CAD build for the part. Positions are in the model's coordinates, mm. A direction names the side the tool comes from. Round coordinates to 2 decimals unless told otherwise and drop trailing zeros. Order: outer loops, then holes, each group sorted by start corner. A loop starts at its lowest first (then second) coordinate and runs counter-clockwise, first axis right, second up. Notation, with made-up numbers: M 58,-16 L 81,-16 A23 cw 81,3 Z; hole C 56,-6.5 d7. An arc over 180 degrees is marked long. Put each result on its own line as item: value.
```python
from build123d import *

# Parameters (mm, degrees)
SKETCH4_W              = 63.5
SKETCH4_H              = 44.45
BASE_FLANGE1_DEPTH     = 1.905
SKETCHED_START         = -31.75
SKETCHED_BEND3_DEPTH   = 63.5
SKETCHED_BEND3_2_DEPTH = 63.5
CUT_EXTRUDE2_REACH     = 44.696
SKETCH20_R             = 2


# Read off the part's stored shape, not the designer's step: Sketched Bend3
# Sheet-metal steps are written as plain solids
with BuildPart() as part:
    # Sketch4 → Base-Flange1 (new body)
    with BuildSketch(Plane(origin=(0, 0, 0), x_dir=(0, 0, -1), z_dir=(1, 0, 0))):
        Rectangle(SKETCH4_W, SKETCH4_H)
    extrude(amount=-BASE_FLANGE1_DEPTH)

    # Sketched Bend3 outline → Sketched Bend3 (cut)
    with BuildSketch(Plane.XY.offset(SKETCHED_START)):
        with BuildLine():
            ThreePointArc((0, -13.357223013), (-1.375727285, -12.406629491), (-1.905, -10.8204))
            Line((-1.905, -10.8204), (-1.905, -22.225))
            Line((-1.905, -22.225), (0, -22.225))
            Line((0, -22.225), (0, -13.357223013))
        make_face()
        with BuildLine():
            Line((-1.905, 22.225), (-1.905, 10.8204))
            ThreePointArc((-1.905, 10.8204), (-1.375727285, 12.406629491), (0, 13.357223013))
            Line((0, 13.357223013), (0, 22.225))
            Line((0, 22.225), (-1.905, 22.225))
        make_face()
    extrude(amount=SKETCHED_BEND3_DEPTH, mode=Mode.SUBTRACT)

    # Sketched Bend3 2 outline → Sketched Bend3 2 (add)
    with BuildSketch(Plane.XY.offset(SKETCHED_START)):
        with BuildLine():
            Line((0, -10.8204), (0, -13.357223013))
            ThreePointArc((0, -13.357223013), (0.364592683, -13.435674577), (0.7366, -13.462))
            Line((0.7366, -13.462), (9.487967924, -13.462))
            Line((9.487967924, -13.462), (9.487967924, -11.557))
            Line((9.487967924, -11.557), (0.7366, -11.557))
            ThreePointArc((0.7366, -11.557), (0.215745145, -11.341254855), (0, -10.8204))
        make_face()
        with BuildLine():
            ThreePointArc((0.7366, 13.462), (0.364592683, 13.435674577), (0, 13.357223013))
            Line((0, 13.357223013), (0, 10.8204))
            ThreePointArc((0, 10.8204), (0.215745145, 11.341254855), (0.7366, 11.557))
            Line((0.7366, 11.557), (9.487967924, 11.557))
            Line((9.487967924, 11.557), (9.487967924, 13.462))
            Line((9.487967924, 13.462), (0.7366, 13.462))
        make_face()
    extrude(amount=SKETCHED_BEND3_2_DEPTH)

    # Cut-Extrude2: up to this face of the body (flat: up to its plane)
    cut_extrude2_end = Plane(part.part.faces().sort_by_distance((5.112283962, -13.462, 0))[0])
    # Sketch20 → Cut-Extrude2 (cut, up to the picked face)
    with BuildSketch(Plane(origin=(0, 13.462, 0), x_dir=(1, 0, 0), z_dir=(0, 1, 0)), mode=Mode.PRIVATE) as cut_extrude2_sk1:
        with Locations(Location((5.08, 0, 0), (0, 0, 180))):
            Circle(SKETCH20_R)
    cut_extrude2_tool1 = split(extrude(cut_extrude2_sk1.sketch, amount=-CUT_EXTRUDE2_REACH, mode=Mode.PRIVATE), bisect_by=cut_extrude2_end, keep=Keep.BOTH, mode=Mode.PRIVATE)
    # Sketch20 → Cut-Extrude2 (cut, up to the picked face)
    with BuildSketch(Plane(origin=(0, 13.462, 0), x_dir=(1, 0, 0), z_dir=(0, 1, 0)), mode=Mode.PRIVATE) as cut_extrude2_sk2:
        with Locations(Location((5.08, 6.35, 0), (0, 0, 180))):
            Circle(SKETCH20_R)
    cut_extrude2_tool2 = split(extrude(cut_extrude2_sk2.sketch, amount=-CUT_EXTRUDE2_REACH, mode=Mode.PRIVATE), bisect_by=cut_extrude2_end, keep=Keep.BOTH, mode=Mode.PRIVATE)
    # Sketch20 → Cut-Extrude2 (cut, up to the picked face)
    with BuildSketch(Plane(origin=(0, 13.462, 0), x_dir=(1, 0, 0), z_dir=(0, 1, 0)), mode=Mode.PRIVATE) as cut_extrude2_sk3:
        with Locations(Location((5.08, 12.7, 0), (0, 0, 180))):
            Circle(SKETCH20_R)
    cut_extrude2_tool3 = split(extrude(cut_extrude2_sk3.sketch, amount=-CUT_EXTRUDE2_REACH, mode=Mode.PRIVATE), bisect_by=cut_extrude2_end, keep=Keep.BOTH, mode=Mode.PRIVATE)
    # Sketch20 → Cut-Extrude2 (cut, up to the picked face)
    with BuildSketch(Plane(origin=(0, 13.462, 0), x_dir=(1, 0, 0), z_dir=(0, 1, 0)), mode=Mode.PRIVATE) as cut_extrude2_sk4:
        with Locations(Location((5.08, 19.05, 0), (0, 0, 180))):
            Circle(SKETCH20_R)
    cut_extrude2_tool4 = split(extrude(cut_extrude2_sk4.sketch, amount=-CUT_EXTRUDE2_REACH, mode=Mode.PRIVATE), bisect_by=cut_extrude2_end, keep=Keep.BOTH, mode=Mode.PRIVATE)
    # Sketch20 → Cut-Extrude2 (cut, up to the picked face)
    with BuildSketch(Plane(origin=(0, 13.462, 0), x_dir=(1, 0, 0), z_dir=(0, 1, 0)), mode=Mode.PRIVATE) as cut_extrude2_sk5:
        with Locations(Location((5.08, -6.35, 0), (0, 0, 180))):
            Circle(SKETCH20_R)
    cut_extrude2_tool5 = split(extrude(cut_extrude2_sk5.sketch, amount=-CUT_EXTRUDE2_REACH, mode=Mode.PRIVATE), bisect_by=cut_extrude2_end, keep=Keep.BOTH, mode=Mode.PRIVATE)
    # Sketch20 → Cut-Extrude2 (cut, up to the picked face)
    with BuildSketch(Plane(origin=(0, 13.462, 0), x_dir=(1, 0, 0), z_dir=(0, 1, 0)), mode=Mode.PRIVATE) as cut_extrude2_sk6:
        with Locations(Location((5.08, -12.7, 0), (0, 0, 180))):
            Circle(SKETCH20_R)
    cut_extrude2_tool6 = split(extrude(cut_extrude2_sk6.sketch, amount=-CUT_EXTRUDE2_REACH, mode=Mode.PRIVATE), bisect_by=cut_extrude2_end, keep=Keep.BOTH, mode=Mode.PRIVATE)
    # Sketch20 → Cut-Extrude2 (cut, up to the picked face)
    with BuildSketch(Plane(origin=(0, 13.462, 0), x_dir=(1, 0, 0), z_dir=(0, 1, 0)), mode=Mode.PRIVATE) as cut_extrude2_sk7:
        with Locations(Location((5.08, -19.05, 0), (0, 0, 180))):
            Circle(SKETCH20_R)
    cut_extrude2_tool7 = split(extrude(cut_extrude2_sk7.sketch, amount=-CUT_EXTRUDE2_REACH, mode=Mode.PRIVATE), bisect_by=cut_extrude2_end, keep=Keep.BOTH, mode=Mode.PRIVATE)
    add(cut_extrude2_tool1.solids().sort_by(Axis((5.08, 13.462, 0), (0, -1, 0)))[0], mode=Mode.SUBTRACT)
    add(cut_extrude2_tool2.solids().sort_by(Axis((5.08, 13.462, -6.35), (0, -1, 0)))[0], mode=Mode.SUBTRACT)
    add(cut_extrude2_tool3.solids().sort_by(Axis((5.08, 13.462, -12.7), (0, -1, 0)))[0], mode=Mode.SUBTRACT)
    add(cut_extrude2_tool4.solids().sort_by(Axis((5.08, 13.462, -19.05), (0, -1, 0)))[0], mode=Mode.SUBTRACT)
    add(cut_extrude2_tool5.solids().sort_by(Axis((5.08, 13.462, 6.35), (0, -1, 0)))[0], mode=Mode.SUBTRACT)
    add(cut_extrude2_tool6.solids().sort_by(Axis((5.08, 13.462, 12.7), (0, -1, 0)))[0], mode=Mode.SUBTRACT)
    add(cut_extrude2_tool7.solids().sort_by(Axis((5.08, 13.462, 19.05), (0, -1, 0)))[0], mode=Mode.SUBTRACT)


solid = part.part
```
Item 1: Band-saw the part on D-D on x = 5.08. State how many separate pieces and enclosed holes the cut face has, and give its area (3 significant figures).
Answers below:
separate pieces: 16
enclosed holes: 0
area: 135 mm²
Item 2: Pin check, flat tip, straight feed: P1, Ø6, axis at y = -6, z = 18, coming from the +X side. Stop position of the tip, or through.
Answers below:
P1: x = 0
Item 3: Mould opens along Y. For faces 3 (the flat face through (2, 11.557, 0)), 4 (the flat face through (8, 13.462, 0)), 5 (the cylindrical face through (3.233, 12.523, 5.584)) say: pulls with the +Y half, pulls with the -Y half, needs draft (parallel to the pull), parting line crosses it, or undercut.
Answers below:
face 3: undercut
face 4: pulls with the +Y half
face 5: needs draft
Item 4: Tool access for faces 1 (the cylindrical face through (4.005, 12.523, -4.664)), 2 (the flat face through (0, 0, 0)): list every direction of +Z, -Z, +X, -X, +Y, -Y with a clear straight run to the whole face (end or side of a thin tool).
Answers below:
face 1: +Y, -Y
face 2: +Z, -Z, +X
Item 5: Band-saw the part on A-A on x = 2. Give the cut face in (y, z), and give its area (3 significant figures).
Answers below:
outline: M -13.46,-31.75 L -11.56,-31.75 L -11.56,31.75 L -13.46,31.75 Z; M 11.56,-31.75 L 13.46,-31.75 L 13.46,31.75 L 11.56,31.75 Z
area: 242 mm²
Item 6: Probe line 1 along Y through (x, z) = (1, 8.5); line 2 along X through (y, z) = (-2.5, -22) (3 decimals); line 3 along Y through (x, z) = (0.5, 19). List the from-to ranges inside material, lowest first. Write a range as [from, to].
Answers below:
line 1: [-13.46, -11.56], [11.56, 13.46]
line 2: [-1.905, 0]
line 3: [-13.45, -11.52], [11.52, 13.45]
Item 7: Band-saw the part on B-B on z = 6.35. Give the cut face in (x, y) (3 decimals), and give its area (3 significant figures).
Answers below:
outline: M -1.905,-10.82 A2.642 ccw 0.737,-13.462 L 3.08,-13.462 L 3.08,-11.557 L 0.737,-11.557 A0.737 cw 0,-10.82 L 0,10.82 A0.737 cw 0.737,11.557 L 3.08,11.557 L 3.08,13.462 L 0.737,13.462 A2.642 ccw -1.905,10.82 Z; M 7.08,-13.462 L 9.488,-13.462 L 9.488,-11.557 L 7.08,-11.557 Z; M 7.08,11.557 L 9.488,11.557 L 9.488,13.462 L 7.08,13.462 Z
area: 69.4 mm²
Item 8: Band-saw the part on C-C on y = 3.75. Give the cut face in (x, z) (3 decimals), and give its area (3 significant figures).
Answers below:
outline: M -1.905,-31.75 L 0,-31.75 L 0,31.75 L -1.905,31.75 Z
area: 121 mm²
